from build123d import *

# Parameters (mm, degrees)
CROQUIS1_W               = 22
CROQUIS1_H               = 55.2
SALIENTE_EXTRUIR1_DEPTH  = 4
CROQUIS2_W               = 12.1
CROQUIS2_H               = 4
CORTAR_EXTRUIR1_DEPTH    = 9.6
CROQUIS3_W               = 12.1
CROQUIS3_H               = 4
CORTAR_EXTRUIR2_DEPTH    = 9.6
CORTAR_EXTRUIR3_DEPTH    = 16
CORTAR_EXTRUIR4_START    = -16
CORTAR_EXTRUIR4_DEPTH    = 16
CROQUIS9_W               = 11.778481694
CROQUIS9_H               = 4
CORTAR_EXTRUIR5_DEPTH    = 2
CROQUIS11_W              = 4.95
CROQUIS11_H              = 4
SALIENTE_EXTRUIR3_DEPTH  = 2
CROQUIS12_W              = 4
CROQUIS12_H              = 1.8
SALIENTE_EXTRUIR4_DEPTH  = 12.1
CROQUIS13_W              = 4.95
CROQUIS13_H              = 4
SALIENTE_EXTRUIR5_DEPTH  = 2
CROQUIS14_W              = 4
CROQUIS14_H              = 1.8
SALIENTE_EXTRUIR6_DEPTH  = 12.1
CROQUIS17_W              = 4
CROQUIS17_H              = 59.2
SALIENTE_EXTRUIR8_DEPTH  = 11.5
CROQUIS18_W              = 4
CROQUIS18_H              = 59.2
SALIENTE_EXTRUIR9_DEPTH  = 11.5
CROQUIS19_R              = 1.75
CORTAR_EXTRUIR6_DEPTH    = 11.5
CORTAR_EXTRUIR7_DEPTH    = 10
CROQUIS27_W              = 12.1
CROQUIS27_H              = 55.6
CORTAR_EXTRUIR8_DEPTH    = 10
CROQUIS28_W              = 12.1
CROQUIS28_H              = 4
SALIENTE_EXTRUIR10_DEPTH = 55.6
SALIENTE_EXTRUIR11_DEPTH = 4.5
CROQUIS30_R              = 2.1
CORTAR_EXTRUIR9_DEPTH    = 10


with BuildPart() as part:
    # Croquis1 → Saliente-Extruir1 (new body)
    with BuildSketch(Plane.XY):
        with Locations((11, 27.6)):
            Rectangle(CROQUIS1_W, CROQUIS1_H)
    extrude(amount=SALIENTE_EXTRUIR1_DEPTH)

    # Croquis2 → Cortar-Extruir1 (cut)
    with BuildSketch(Plane(origin=(0, 55.2, 0), x_dir=(1, 0, 0), z_dir=(0, 1, 0))):
        with Locations((11, -2)):
            Rectangle(CROQUIS2_W, CROQUIS2_H)
    extrude(amount=-CORTAR_EXTRUIR1_DEPTH, mode=Mode.SUBTRACT)

    # Croquis3 → Cortar-Extruir2 (cut)
    with BuildSketch(Plane.XZ):
        with Locations((11, 2)):
            Rectangle(CROQUIS3_W, CROQUIS3_H)
    extrude(amount=-CORTAR_EXTRUIR2_DEPTH, mode=Mode.SUBTRACT)

    # Croquis5 → Cortar-Extruir3 (cut)
    with BuildSketch(Plane.XZ.offset(-9.6)):
        with BuildLine():
            Line((7.4, 4), (14.6, 4))
            ThreePointArc((14.6, 4), (16.401151853, 1.506649462), (17.05, -1.5))
            Line((17.05, -1.5), (4.95, -1.5))
            ThreePointArc((4.95, -1.5), (5.598848147, 1.506649462), (7.4, 4))
        make_face()
    extrude(amount=-CORTAR_EXTRUIR3_DEPTH, mode=Mode.SUBTRACT)

    # Croquis7 → Cortar-Extruir4 (cut)
    with BuildSketch(Plane(origin=(0, 45.6, 0), x_dir=(1, 0, 0), z_dir=(0, 1, 0)).offset(CORTAR_EXTRUIR4_START)):
        with BuildLine():
            Line((4.95, 1.5), (17.05, 1.5))
            ThreePointArc((17.05, 1.5), (16.401151853, -1.506649462), (14.6, -4))
            Line((14.6, -4), (7.4, -4))
            ThreePointArc((7.4, -4), (5.598848147, -1.506649462), (4.95, 1.5))
        make_face()
    extrude(amount=CORTAR_EXTRUIR4_DEPTH, mode=Mode.SUBTRACT)

    # Croquis9 → Cortar-Extruir5 (cut)
    with BuildSketch(Plane(origin=(0, 0, 0), x_dir=(-1, 0, 0), z_dir=(0, 0, -1))):
        with Locations((-11, 27.6)):
            Rectangle(CROQUIS9_W, CROQUIS9_H)
    extrude(amount=-CORTAR_EXTRUIR5_DEPTH, mode=Mode.SUBTRACT)

    # Croquis11 → Saliente-Extruir3 (add)
    with BuildSketch(Plane(origin=(0, 55.2, 0), x_dir=(1, 0, 0), z_dir=(0, 1, 0))):
        with Locations((2.475, -2)):
            Rectangle(CROQUIS11_W, CROQUIS11_H)
        with Locations((19.525, -2)):
            Rectangle(CROQUIS11_W, CROQUIS11_H)
    extrude(amount=SALIENTE_EXTRUIR3_DEPTH)

    # Croquis12 → Saliente-Extruir4 (add)
    with BuildSketch(Plane(origin=(4.95, 0, 0), x_dir=(0, 0, -1), z_dir=(1, 0, 0))):
        with Locations((-2, 56.3)):
            Rectangle(CROQUIS12_W, CROQUIS12_H)
    extrude(amount=SALIENTE_EXTRUIR4_DEPTH)

    # Croquis13 → Saliente-Extruir5 (add)
    with BuildSketch(Plane.XZ):
        with Locations((19.525, 2)):
            Rectangle(CROQUIS13_W, CROQUIS13_H)
        with Locations((2.475, 2)):
            Rectangle(CROQUIS13_W, CROQUIS13_H)
    extrude(amount=SALIENTE_EXTRUIR5_DEPTH)

    # Croquis14 → Saliente-Extruir6 (add)
    with BuildSketch(Plane(origin=(4.95, 0, 0), x_dir=(0, 0, -1), z_dir=(1, 0, 0))):
        with Locations((-2, -1.1)):
            Rectangle(CROQUIS14_W, CROQUIS14_H)
    extrude(amount=SALIENTE_EXTRUIR6_DEPTH)

    # Croquis17 → Saliente-Extruir8 (add)
    with BuildSketch(Plane.ZY):
        with Locations((2, 27.6)):
            Rectangle(CROQUIS17_W, CROQUIS17_H)
    extrude(amount=SALIENTE_EXTRUIR8_DEPTH)

    # Croquis18 → Saliente-Extruir9 (add)
    with BuildSketch(Plane(origin=(22, 0, 0), x_dir=(0, 0, -1), z_dir=(1, 0, 0))):
        with Locations((-2, 27.6)):
            Rectangle(CROQUIS18_W, CROQUIS18_H)
    extrude(amount=SALIENTE_EXTRUIR9_DEPTH)

    # Croquis19 → Cortar-Extruir6 (cut)
    with BuildSketch(Plane(origin=(0, 0, 0), x_dir=(-1, 0, 0), z_dir=(0, 0, -1))):
        with Locations((-23.2, 54)):
            Circle(CROQUIS19_R)
        with Locations((1.2, 54.8)):
            Circle(CROQUIS19_R)
        with Locations((1.2, 0.5)):
            Circle(CROQUIS19_R)
        with Locations((-23.2, 0.5)):
            Circle(CROQUIS19_R)
    extrude(amount=-CORTAR_EXTRUIR6_DEPTH, mode=Mode.SUBTRACT)

    # Croquis21 → Cortar-Extruir7 (cut)
    with BuildSketch(Plane(origin=(0, 0, 0), x_dir=(-1, 0, 0), z_dir=(0, 0, -1))):
        Polygon((-27.345452568, 57.2), (-33.5, 32.755874525), (-33.5, 57.2), align=None)
        Polygon((4.445660904, 57.2), (11.5, 32.755874525), (11.5, 57.2), align=None)
        Polygon((-25.363668871, -2), (-33.5, 23.094679002), (-33.5, -2), align=None)
        Polygon((11.5, 23.094679002), (5.766850036, -2), (11.5, -2), align=None)
    extrude(amount=-CORTAR_EXTRUIR7_DEPTH, mode=Mode.SUBTRACT)

    # Croquis27 → Cortar-Extruir8 (cut)
    with BuildSketch(Plane(origin=(0, 0, 0), x_dir=(-1, 0, 0), z_dir=(0, 0, -1))):
        with Locations((-11, 27.6)):
            Rectangle(CROQUIS27_W, CROQUIS27_H)
    extrude(amount=-CORTAR_EXTRUIR8_DEPTH, mode=Mode.SUBTRACT)

    # Croquis28 → Saliente-Extruir10 (add)
    with BuildSketch(Plane.XZ.offset(-55.4)):
        with Locations((11, 2)):
            Rectangle(CROQUIS28_W, CROQUIS28_H)
    extrude(amount=SALIENTE_EXTRUIR10_DEPTH)

    # Croquis29 → Saliente-Extruir11 (add)
    with BuildSketch(Plane(origin=(0, 0, 0), x_dir=(-1, 0, 0), z_dir=(0, 0, -1))):
        with BuildLine():
            Line((-21.25, 32.527178544), (-21.25, 23.323374983))
            ThreePointArc((-21.25, 23.323374983), (-31.1, 27.925276764), (-21.25, 32.527178544))
        make_face()
        with BuildLine():
            Line((-1.112987938, 23.653189144), (-1.112987938, 32.197364384))
            ThreePointArc((-1.112987938, 32.197364384), (9.1, 27.925276764), (-1.112987938, 23.653189144))
        make_face()
    extrude(amount=SALIENTE_EXTRUIR11_DEPTH)

    # Croquis25 → Cortar-Revolución3 (revolve, cut)
    with BuildSketch(Plane(origin=(0, 0, -7.5), x_dir=(-1, 0, 0), z_dir=(0, 0, -1))):
        with BuildLine():
            Line((-25.1, 22.925276764), (-25.1, 32.925276764))
            ThreePointArc((-25.1, 32.925276764), (-30.1, 27.925276764), (-25.1, 22.925276764))
        make_face()
    revolve(axis=Axis((25.1, 22.925276764, -7.5), (0, 1, 0)), mode=Mode.SUBTRACT)

    # Croquis26 → Cortar-Revolución4 (revolve, cut)
    with BuildSketch(Plane(origin=(0, 0, -7.5), x_dir=(-1, 0, 0), z_dir=(0, 0, -1))):
        with BuildLine():
            Line((3.1, 32.925276764), (3.1, 22.925276764))
            ThreePointArc((3.1, 22.925276764), (8.1, 27.925276764), (3.1, 32.925276764))
        make_face()
    revolve(axis=Axis((-3.1, 32.925276764, -7.5), (0, -1, 0)), mode=Mode.SUBTRACT)

    # Croquis30 → Cortar-Extruir9 (cut)
    with BuildSketch(Plane(origin=(0, 0, 0), x_dir=(-1, 0, 0), z_dir=(0, 0, -1))):
        with Locations((-25.1, 37.194789274)):
            Circle(CROQUIS30_R)
        with Locations((-25.1, 16.925277734)):
            Circle(CROQUIS30_R)
        with Locations((3.1, 37.194789274)):
            Circle(CROQUIS30_R)
        with Locations((3.1, 16.925277734)):
            Circle(CROQUIS30_R)
    extrude(amount=-CORTAR_EXTRUIR9_DEPTH, mode=Mode.SUBTRACT)


solid = part.part
Input: part model. Units: mm. Frame: model coordinates. A direction names the side the tool comes from. Round coordinates to 2 decimals unless told otherwise and drop trailing zeros. Write each loop counter-clockwise with the first axis right and the second up, starting at its lowest first coordinate (ties: lowest second). Pieces come first, ordered by that corner, then holes.
1) Cut plane C-C (x = 2.5). Return the cut outline in (y, z).
2) Contact query for flat-ended pins moving along their axis: P1, Ø10, axis at x = 3.5, y = 32.5, coming from the -Z side; P2, Ø3.5, axis at x = -3.1, y = 37.19, coming from the -Z side; P3, Ø1, axis at x = 22.5, y = 4.5, coming from the -Z side; P4, Ø1, axis at y = 24, z = -1.5, coming from the +X side. Output: stop coordinate, or through.
3) Reachability of faces 5 (the flat face through (-8.674, 10.723, 1.972)), 6 (the cylindrical face through (-9.097, 28.123, -2.218)), 7 (the flat face through (1.113, 28, -2)) from +Z, -Z, +X, -X, +Y, -Y: full face, straight path, thin tool, end or side. Return the list, or none.
4) Draft query along Y for faces 1 (the cylindrical face through (-2.817, -0.17, 1.972)), 2 (the cylindrical face through (21.531, 1.026, 1.972)), 3 (the flat face through (-7.923, 45.149, 1.972)), 4 (the cylindrical face through (31.097, 27.735, -2.218)). Return one class per face: pulls with the +Y half, pulls with the -Y half, needs draft (parallel to the pull), parting line crosses it, or undercut.
5) Cut plane D-D (z = 1.75). Count the separate pieces of the cut face and the enclosed holes in it, then the cut area to 3 significant figures.
6) Ray query, L1, parallel to Y at x = -1.2, z = 2; L2, parallel to Y at x = 23.2, z = 3.1; L3, parallel to Z at x = 30, y = 22. Return the intervals inside material, ascending.
7) Cut plane B-B (z = -3.5). Return the cut outline in (x, y), then the cut area to 3 significant figures.
8) Cut plane A-A (y = 54). Return the cut outline in (x, z).
Geometry says:
1. outline: (-2, 0) - (57.2, 0) - (57.2, 4) - (-2, 4) - close
2. P1: stops at z = -4.5
2. P2: passes through
2. P3: stops at z = 0
2. P4: stops at x = 30.03
3. face 5: +Z, -Z, -X, -Y
3. face 6: -Z
3. face 7: -Z, +Y, -Y
4. face 1: undercut
4. face 2: undercut
4. face 3: pulls with the +Y half
4. face 4: parting line crosses it
5. separate pieces: 1
5. enclosed holes: 8
5. area: 2,230 mm2
6. L1: y = -2 to -1.25, 2.25 to 16.03, 17.82 to 36.3, 38.09 to 53.05, 56.55 to 57.2
6. L2: y = -2 to -1.25, 2.25 to 16.03, 17.82 to 36.3, 38.09 to 52.25, 55.75 to 57.2
6. L3: z = 0 to 4
7. outline: (1.11, 23.65) - (1.11, 32.2) arc R6 ccw (long way) to start; (21.25, 23.32) arc R6 ccw (long way) to (21.25, 32.53) - close; hole circle Ø6 at (-3.1, 27.93); hole circle Ø6 at (25.1, 27.93)
7. area: 145 mm2
8. outline: (-5.37, 0) - (-2.76, 0) - (-2.76, 4) - (-5.37, 4) - close; (0.36, 0) - (21.45, 0) - (21.45, 4) - (0.36, 4) - close; (24.95, 0) - (28.15, 0) - (28.15, 4) - (24.95, 4) - close
